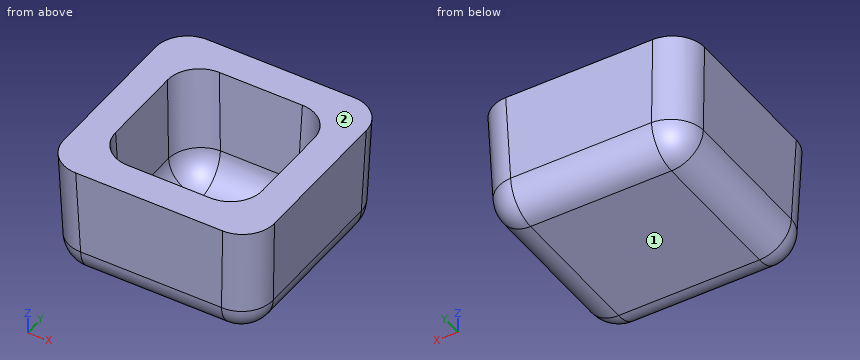
```python
from build123d import *

# Parameters (mm, degrees)
F0_W     = 66
F0_H     = 66
F0_W_2   = 46
F0_H_2   = 46
F1_DEPTH = 37
F1_TAPER = 2
F2_DEPTH = 35.5
F2_TAPER = 2
F3_R     = 10
F4_R     = 10


with BuildPart() as f1:
    # F0 (on Top) → F1 (new body)
    with BuildSketch(Plane.XY):
        with Locations((33, 33)):
            Rectangle(F0_W, F0_H)
        with Locations((33, 33)):
            Rectangle(F0_W_2, F0_H_2, mode=Mode.SUBTRACT)
        with Locations((33, 33)):
            Rectangle(F0_W_2, F0_H_2)
    extrude(amount=-F1_DEPTH, taper=F1_TAPER)

    # F0 (on Top) → F2 (cut)
    with BuildSketch(Plane.XY):
        with Locations((33, 33)):
            Rectangle(F0_W_2, F0_H_2)
    extrude(amount=-F2_DEPTH, taper=F2_TAPER, mode=Mode.SUBTRACT)

    # F3
    f3_edges = [f1.edges().sort_by_distance(p)[0] for p in [
        (11.239687, 33, -35.5),
        (33, 11.239687, -35.5),
        (54.760313, 33, -35.5),
        (33, 54.760313, -35.5),
        (55.380156, 10.619844, -17.75),
        (10.619844, 55.380156, -17.75),
        (10.619844, 10.619844, -17.75),
        (55.380156, 55.380156, -17.75),
    ]]
    fillet(f3_edges, radius=F3_R)

    # F4
    f4_edges = [f1.edges().sort_by_distance(p)[0] for p in [
        (1.292068, 33, -37),
        (33, 1.292068, -37),
        (64.707932, 33, -37),
        (33, 64.707932, -37),
        (65.353966, 65.353966, -18.5),
        (0.646034, 65.353966, -18.5),
        (0.646034, 0.646034, -18.5),
        (65.353966, 0.646034, -18.5),
    ]]
    fillet(f4_edges, radius=F4_R)


solid = f1.part
```
The listing builds one solid part. Answer for the finished solid, in the listing's coordinates (mm). Face numbers are marked on the shaded views. Round coordinates to 2 decimals unless told otherwise and drop trailing zeros.
Q1. Find the intervals of material crossed by line 1 (X direction, y = 24, z = -14.5); line 2 (Z direction, x = 34, y = 28); line 3 (Y direction, x = 30, z = -18), in increasing order.
Q2. Given pin 1 Ø3 at (x, z) = (35, -9) entering from +Y; pin 2 Ø10 at (x, z) = (25.5, -5) entering from -Y; pin 3 Ø4 at (x, z) = (54.5, -16) entering from +Y; pin 4 Ø2 at (y, z) = (48, -19) entering from -X, each flat-ended and moving along its own axis, determine where each tip first touches the part or whether it passes through.
Q3. For a pull along Z with two mould halves and no side action, classify the marked faces 1 and 2 as released by +Z, released by -Z, zero draft, split by the parting line, or undercut.
Completed:
1. line 1: x = 0.51 to 10.51, 55.49 to 65.49
1. line 2: z = -37 to -35.5
1. line 3: y = 0.63 to 10.63, 55.37 to 65.37
2. pin 1: stops at y = 65.74
2. pin 2: stops at y = 0
2. pin 3: stops at y = 65.51
2. pin 4: stops at x = 0.63
3. face 1: released by -Z
3. face 2: released by +Z
